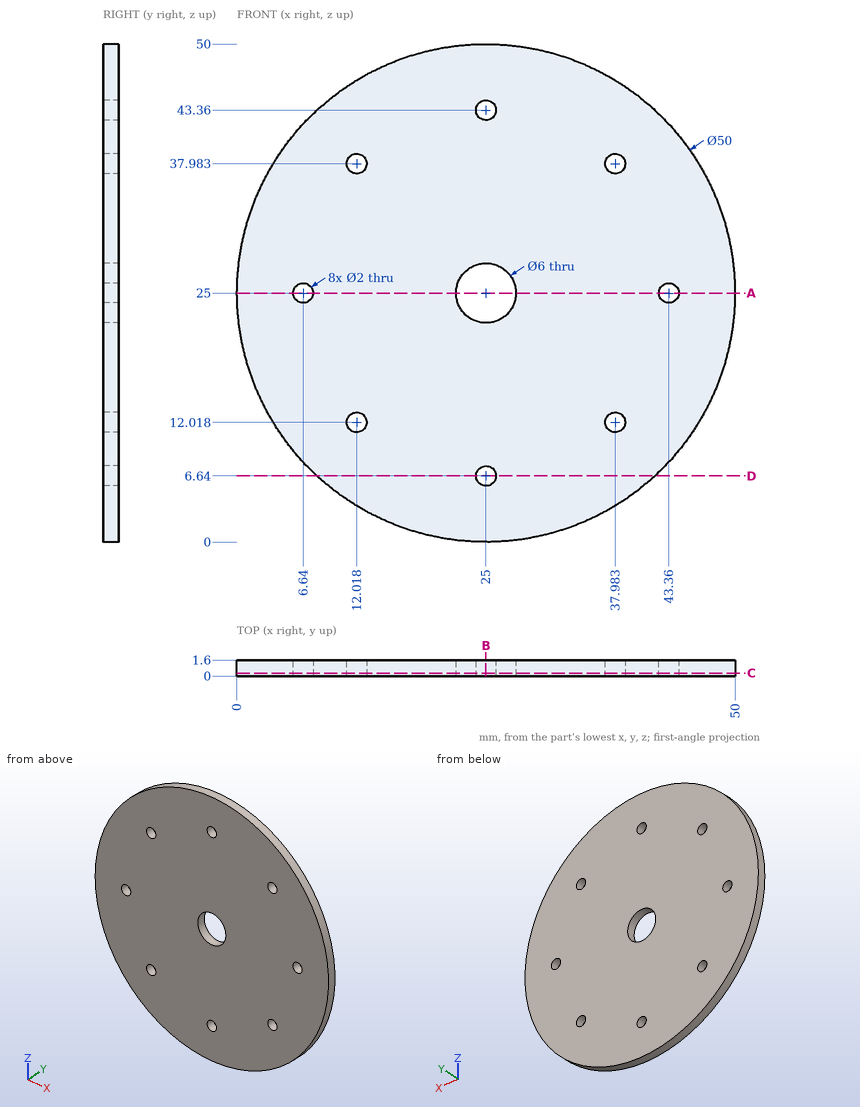
The figure shows three views and two pictorial views of one solid part (mm, origin at its lowest corner). Answer the questions. Give positions to 0.01 mm unless a question says otherwise; leave off trailing zeros. Order: outer loops, then holes, each group sorted by start corner. A loop starts at its lowest first (then second) coordinate and runs counter-clockwise, first axis right, second up. Notation, with made-up numbers: M 31.5,88.25 L 42.5,88.25 A26 cw 42.5,102.25 Z; hole C -9,41 d2. An arc over 180 degrees is marked long. Return JSON: item names as keys, results as strings.
Q1. Find section A-A, the plane z = 25. Write down the section's boundary in (x, y).
Answer below:
{"outline": "M 0,0 L 5.64,0 L 5.64,1.6 L 0,1.6 Z; M 7.64,0 L 22,0 L 22,1.6 L 7.64,1.6 Z; M 28,0 L 42.36,0 L 42.36,1.6 L 28,1.6 Z; M 44.36,0 L 50,0 L 50,1.6 L 44.36,1.6 Z"}
Q2. Find section D-D, the plane z = 6.64. Write down the section's boundary in (x, y).
Answer below:
{"outline": "M 8.03,0 L 24,0 L 24,1.6 L 8.03,1.6 Z; M 26,0 L 41.97,0 L 41.97,1.6 L 26,1.6 Z"}
Q3. Find section C-C, the plane y = 0.3. State how many separate pieces and enclosed holes the cut face has, and give its area (3 significant figures).
Answer below:
{"separate pieces": "1", "enclosed holes": "9", "area": "1,910 mm^2"}
Q4. This flat-tipped pin is pushed along its axis until it touches: pin 1 (5.5 mm diameter, centred on x = 25, z = 25, fed in from -Y). Where does it stop, or does it pass through?
Answer below:
{"pin 1": "passes through"}
Q5. Find section B-B, the plane x = 25. Write down the section's boundary in (y, z).
Answer below:
{"outline": "M 0,0 L 1.6,0 L 1.6,5.64 L 0,5.64 Z; M 0,7.64 L 1.6,7.64 L 1.6,22 L 0,22 Z; M 0,28 L 1.6,28 L 1.6,42.36 L 0,42.36 Z; M 0,44.36 L 1.6,44.36 L 1.6,50 L 0,50 Z"}
Q6. Find the intervals of material crossed by line 1 along X through (y, z) = (1.35, 25.5) (1 decimal); line 2 along X through (y, z) = (1.45, 38) (1 decimal); line 3 along X through (y, z) = (0.2, 43.5) (1 decimal), in increasing order. Write a range as [from, to].
Answer below:
{"line 1": "x = [0, 5.8], [7.5, 22], [28, 42.5], [44.2, 50]", "line 2": "x = [3.6, 11], [13, 37], [39, 46.4]", "line 3": "x = [8.2, 24], [26, 41.8]"}
